from build123d import *

# Parameters (mm, degrees)
EXTRUDE_1_DEPTH     = 7
SKETCH_2_R          = 4.1
SKETCH_2_R_2        = 1.25
SKETCH_2_R_3        = 4
CUT_EXTRUDE_1_DEPTH = 10
SKETCH_3_R          = 11
CUT_EXTRUDE_2_DEPTH = 2.5
SKETCH_7_R          = 4.1
EXTRUDE_4_DEPTH     = 7
SKETCH_13_R         = 1.75
CUT_EXTRUDE_3_DEPTH = 10
SKETCH_15_R         = 4.01
CUT_EXTRUDE_5_DEPTH = 3


with BuildPart() as part:
    # 草图1 → 凸台-拉伸1 (new body)
    with BuildSketch(Plane.XY):
        with BuildLine():
            Line((0, -10), (90, -18))
            ThreePointArc((90, -18), (105, -3), (90, 12))
            Line((90, 12), (0, 10))
            ThreePointArc((0, 10), (-10, 0), (0, -10))
        make_face()
    extrude(amount=EXTRUDE_1_DEPTH)

    # 草图2 → 切除-拉伸1 (cut)
    with BuildSketch(Plane(origin=(0, 0, 0), x_dir=(-1, 0, 0), z_dir=(0, 0, -1))):
        Circle(SKETCH_2_R)
        with Locations((-90, -10)):
            Circle(SKETCH_2_R_2)
        with Locations((-83, -3)):
            Circle(SKETCH_2_R_2)
        with Locations((-90, 4)):
            Circle(SKETCH_2_R_2)
        with Locations((-97, -3)):
            Circle(SKETCH_2_R_2)
        with Locations((-90, -3)):
            Circle(SKETCH_2_R_3)
    extrude(amount=-CUT_EXTRUDE_1_DEPTH, mode=Mode.SUBTRACT)

    # 草图3 → 切除-拉伸2 (cut)
    with BuildSketch(Plane.XY.offset(7)):
        with Locations((90, -3)):
            Circle(SKETCH_3_R)
    extrude(amount=-CUT_EXTRUDE_2_DEPTH, mode=Mode.SUBTRACT)

    # 草图7 → 凸台-拉伸4 (add)
    with BuildSketch(Plane(origin=(0, 0, 0), x_dir=(-1, 0, 0), z_dir=(0, 0, -1))):
        Circle(SKETCH_7_R)
    extrude(amount=-EXTRUDE_4_DEPTH)

    # 草图13 → 切除-拉伸3 (cut)
    with BuildSketch(Plane.XY.offset(7)):
        Circle(SKETCH_13_R)
    extrude(amount=-CUT_EXTRUDE_3_DEPTH, mode=Mode.SUBTRACT)

    # 草图15 → 切除-拉伸5 (cut)
    with BuildSketch(Plane(origin=(0, 0, 0), x_dir=(-1, 0, 0), z_dir=(0, 0, -1))):
        Circle(SKETCH_15_R)
    extrude(amount=-CUT_EXTRUDE_5_DEPTH, mode=Mode.SUBTRACT)


solid = part.part
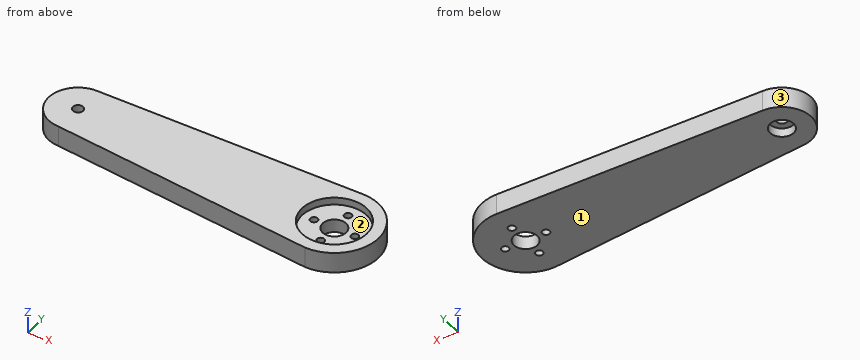
Can you work these out from the model? Positions are in its coordinate system, mm. Face numbers are marked on the shaded views. Coordinates: 2 decimals unless noted, no trailing zeros. Order: outer loops, then holes, each group sorted by start corner. A loop starts at its lowest first (then second) coordinate and runs counter-clockwise, first axis right, second up. Notation, with made-up numbers: (44, 45.25) -> (73, 45.25) arc R24 ccw to (73, 81.25) -> close; hole circle Ø6 at (89.5, -32). An arc over 180 degrees is marked (long way). Use one line per item in the form item = value.
Q1. Imagine slicing it at D-D, the plane y = 6.5. List the corners of the cut face in (x, z) for me.
From the geometry:
outline = (-7.6, 0) -> (101.61, 0) -> (101.61, 7) -> (95.55, 7) -> (95.55, 4.5) -> (84.45, 4.5) -> (84.45, 7) -> (-7.6, 7) -> close
Q2. Will these pins go through, and if not, where does the flat tip stop? P1, Ø2, axis at x = 25.5, z = 2, coming from the -Y side; P2, Ø4, axis at x = 0, y = 0, coming from the -Z side; P3, Ø1, axis at y = -5, z = 3.5, coming from the +X side.
From the geometry:
P1 = -12.36
P2 = 3
P3 = 104.92
Q3. We'd pull the mould along Y, two halves only. Please class the marked faces 1, 2 and 3: released by +Y, released by -Y, zero draft, split by the parting line, or undercut.
From the geometry:
face_1 = zero draft
face_2 = undercut
face_3 = split by the parting line
Q4. Imagine slicing it at C-C, the plane y = -3. List the corners of the cut face in (x, z) for me, then the cut area to 3 significant figures.
From the geometry:
outline = (-9.54, 0) -> (-2.66, 0) -> (-2.66, 3) -> (2.66, 3) -> (2.66, 0) -> (81.75, 0) -> (81.75, 4.5) -> (79, 4.5) -> (79, 7) -> (-9.54, 7) -> close; (84.25, 0) -> (86, 0) -> (86, 4.5) -> (84.25, 4.5) -> close; (94, 0) -> (95.75, 0) -> (95.75, 4.5) -> (94, 4.5) -> close; (98.25, 0) -> (105, 0) -> (105, 7) -> (101, 7) -> (101, 4.5) -> (98.25, 4.5) -> close
area = 672 mm²
Q5. Imagine slicing it at B-B, the plane x = 92.5. List the corners of the cut face in (y, z) for me, then the cut area to 3 significant figures.
From the geometry:
outline = (-17.79, 0) -> (-6.12, 0) -> (-6.12, 4.5) -> (-13.71, 4.5) -> (-13.71, 7) -> (-17.79, 7) -> close; (0.12, 0) -> (11.79, 0) -> (11.79, 7) -> (7.71, 7) -> (7.71, 4.5) -> (0.12, 4.5) -> close
area = 125 mm²
Q6. I need wall thicknesses on L1, parallel to Y at x = 90, z = 2.7; L2, parallel to Y at x = 0, z = 5.1; L3, parallel to Z at x = 97, y = 5. Which ranges of each line are inside material? Lowest first, please.
From the geometry:
L1 = -18 to -11.25, -8.75 to -7, 1 to 2.75, 5.25 to 12
L2 = -10 to -1.75, 1.75 to 10
L3 = 0 to 4.5
Q7. Imagine slicing it at A-A, the plane z = 5.75. List the corners of the cut face in (x, y) for me.
From the geometry:
outline = (0, -10) -> (90, -18) arc R15 ccw to (90, 12) -> (0, 10) arc R10 ccw to start; hole circle Ø3.5 at (0, 0); hole circle Ø22 at (90, -3)
